Read the model definition and answer for the solid it produces. Units are mm, in the model's axes. Face numbers are marked on the shaded views. Round coordinates to 2 decimals unless told otherwise and drop trailing zeros. Answer as CSV lines item,"result".
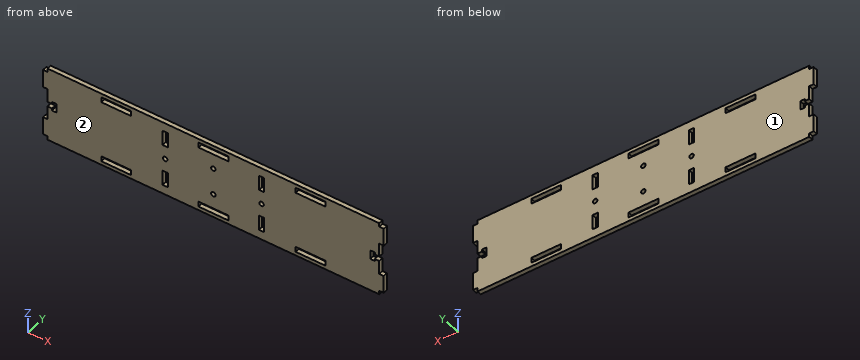
```python
from build123d import *

# Parameters (mm, degrees)
CROQUIS1_R              = 1.5
CROQUIS1_W              = 20
CROQUIS1_H              = 3.5
CROQUIS1_W_2            = 3.5
CROQUIS1_H_2            = 10
SALIENTE_EXTRUIR1_DEPTH = 3
CROQUIS2_W              = 11.85
CROQUIS2_H              = 3
CROQUIS2_W_2            = 12
SALIENTE_EXTRUIR2_DEPTH = 3


with BuildPart() as part:
    # Croquis1 → Saliente-Extruir1 (new body)
    with BuildSketch(Plane(origin=(0, 0, 0), x_dir=(1, 0, 0), z_dir=(0, 1, 0))):
        Polygon((111, -25), (-111, -25), (-111, -1.55), (-108, -1.55), (-108, -3), (-105, -3), (-105, 3), (-108, 3), (-108, 1.55), (-111, 1.55), (-111, 25), (111, 25), (111, 1.55), (108, 1.55), (108, 3), (105, 3), (105, -3), (108, -3), (108, -1.55), (111, -1.55), align=None)
        with Locations(Location((-32.25, 0, 0), (0, 0, 270))):
            Circle(CROQUIS1_R, mode=Mode.SUBTRACT)
        with Locations(Location((32.25, 0, 0), (0, 0, 90))):
            Circle(CROQUIS1_R, mode=Mode.SUBTRACT)
        with Locations(Location((0, -9, 0), (0, 0, 270))):
            Circle(CROQUIS1_R, mode=Mode.SUBTRACT)
        with Locations(Location((0, 9, 0), (0, 0, 90))):
            Circle(CROQUIS1_R, mode=Mode.SUBTRACT)
        with Locations((65, 20.75)):
            Rectangle(CROQUIS1_W, CROQUIS1_H, mode=Mode.SUBTRACT)
        with Locations((0, 20.75)):
            Rectangle(CROQUIS1_W, CROQUIS1_H, mode=Mode.SUBTRACT)
        with Locations((-65, 20.75)):
            Rectangle(CROQUIS1_W, CROQUIS1_H, mode=Mode.SUBTRACT)
        with Locations((65, -20.75)):
            Rectangle(CROQUIS1_W, CROQUIS1_H, mode=Mode.SUBTRACT)
        with Locations((0, -20.75)):
            Rectangle(CROQUIS1_W, CROQUIS1_H, mode=Mode.SUBTRACT)
        with Locations((-65, -20.75)):
            Rectangle(CROQUIS1_W, CROQUIS1_H, mode=Mode.SUBTRACT)
        with Locations((-32.25, 14)):
            Rectangle(CROQUIS1_W_2, CROQUIS1_H_2, mode=Mode.SUBTRACT)
        with Locations((-32.25, -14)):
            Rectangle(CROQUIS1_W_2, CROQUIS1_H_2, mode=Mode.SUBTRACT)
        with Locations((32.25, 14)):
            Rectangle(CROQUIS1_W_2, CROQUIS1_H_2, mode=Mode.SUBTRACT)
        with Locations((32.25, -14)):
            Rectangle(CROQUIS1_W_2, CROQUIS1_H_2, mode=Mode.SUBTRACT)
    extrude(amount=SALIENTE_EXTRUIR1_DEPTH)

    # Croquis2 → Saliente-Extruir2 (add)
    with BuildSketch(Plane.ZY.offset(111)):
        with Locations((-16.575, 1.5)):
            Rectangle(CROQUIS2_W, CROQUIS2_H)
        with Locations((16.575, 1.5)):
            Rectangle(CROQUIS2_W_2, CROQUIS2_H)
    saliente_extruir2 = extrude(amount=SALIENTE_EXTRUIR2_DEPTH)

    # Simetría1: Saliente-Extruir2 across plane
    add(saliente_extruir2.mirror(Plane(origin=(0, 0, 0), x_dir=(0, 0, 1), z_dir=(1, 0, 0))))


solid = part.part
```
1) Determine the mould class of the marked faces 1 and 2 for opening direction Y: released by +Y, released by -Y, zero draft, split by the parting line, or undercut.
Evaluation:
face 1,"released by +Y"
face 2,"released by -Y"
2) Each of these flat-tipped pins is pushed along its axis until it touches: P1, Ø0.9, axis at y = 1, z = 5.5, coming from the -X side; P2, Ø1.5, axis at y = 2.5, z = 3.5, coming from the +X side. Where does it stop, or does it pass through?
Evaluation:
P1,"stops at x = -111"
P2,"stops at x = 111"
3) Find section A-A, the plane y = 1.2. Count the separate pieces of the cut face and the enclosed holes in it, then the cut area to 3 significant figures.
Evaluation:
separate pieces,"1"
enclosed holes,"14"
area,"10,600 mm^2"
4) Straight lines are drawn through the part: line 1 (Z direction, x = 3, y = 1.6); line 2 (X direction, y = 1.8, z = 22); line 3 (X direction, y = 1.5, z = 0). For each, find the intervals that lie inside material, in ascending order.
Evaluation:
line 1,"z = -25 to -22.5, -19 to 19, 22.5 to 25"
line 2,"x = -114 to -75, -55 to -10, 10 to 55, 75 to 114"
line 3,"x = -105 to -33.75, -30.75 to 30.75, 33.75 to 105"
